from build123d import *

# Parameters (mm, degrees)
SKETCH1_W           = 13
SKETCH1_H           = 23
BOSS_EXTRUDE1_DEPTH = 23
CUT_EXTRUDE1_REACH  = 25
SKETCH1_3_W         = 12
SKETCH1_3_H         = 22
SKETCH2_W           = 13
SKETCH2_H           = 5.5
SKETCH2_R           = 1
BOSS_EXTRUDE2_DEPTH = 1
SKETCH4_W           = 8
SKETCH4_H           = 16
BOSS_EXTRUDE3_DEPTH = 10
CUT_EXTRUDE2_REACH  = 12.5
SKETCH5_W           = 14
SKETCH5_H           = 8
CUT_EXTRUDE3_REACH  = 22
SKETCH6_W           = 7
SKETCH6_H           = 9


with BuildPart() as part:
    # Sketch1 → Boss-Extrude1 (new body)
    with BuildSketch(Plane.XY):
        Rectangle(SKETCH1_W, SKETCH1_H)
    extrude(amount=BOSS_EXTRUDE1_DEPTH)

    # Sketch1_3 → Cut-Extrude1 (cut, up to next)
    with BuildSketch(Plane.XY, mode=Mode.PRIVATE) as cut_extrude1_sk1:
        Rectangle(SKETCH1_3_W, SKETCH1_3_H)
    cut_extrude1_tool1 = extrude(cut_extrude1_sk1.sketch, amount=CUT_EXTRUDE1_REACH, mode=Mode.PRIVATE) & part.part
    add(cut_extrude1_tool1.solids().sort_by_distance((0, 0, 0))[0], mode=Mode.SUBTRACT)

    # Sketch2 → Boss-Extrude2 (add)
    with BuildSketch(Plane.XY.offset(23)):
        with Locations((0, 14.25)):
            Rectangle(SKETCH2_W, SKETCH2_H)
        with Locations((0, 14.5)):
            Circle(SKETCH2_R, mode=Mode.SUBTRACT)
        with Locations((0, -14.25)):
            Rectangle(SKETCH2_W, SKETCH2_H)
        with Locations((0, -14.5)):
            Circle(SKETCH2_R, mode=Mode.SUBTRACT)
    extrude(amount=-BOSS_EXTRUDE2_DEPTH)

    # Sketch4 → Boss-Extrude3 (add)
    with BuildSketch(Plane(origin=(0, -11.5, 0), x_dir=(-1, 0, 0), z_dir=(0, -1, 0))):
        with Locations((0, -11)):
            Rectangle(SKETCH4_W, SKETCH4_H)
    extrude(amount=BOSS_EXTRUDE3_DEPTH)

    # Sketch5 → Cut-Extrude2 (cut, up to next)
    with BuildSketch(Plane(origin=(4, 0, 0), x_dir=(0, 0, -1), z_dir=(1, 0, 0)), mode=Mode.PRIVATE) as cut_extrude2_sk1:
        with Locations((-11, -16.5)):
            Rectangle(SKETCH5_W, SKETCH5_H)
    cut_extrude2_tool1 = extrude(cut_extrude2_sk1.sketch, amount=-CUT_EXTRUDE2_REACH, mode=Mode.PRIVATE) & part.part
    add(cut_extrude2_tool1.solids().sort_by_distance((4, -16.5, 11))[0], mode=Mode.SUBTRACT)

    # Sketch6 → Cut-Extrude3 (cut, up to next)
    with BuildSketch(Plane(origin=(0, 0, 3), x_dir=(-1, 0, 0), z_dir=(0, 0, -1)), mode=Mode.PRIVATE) as cut_extrude3_sk1:
        with Locations((0, -16.5)):
            Rectangle(SKETCH6_W, SKETCH6_H)
    cut_extrude3_tool1 = extrude(cut_extrude3_sk1.sketch, amount=-CUT_EXTRUDE3_REACH, mode=Mode.PRIVATE) & part.part
    add(cut_extrude3_tool1.solids().sort_by_distance((0, -16.5, 3))[0], mode=Mode.SUBTRACT)


solid = part.part
CAD build for the part. Positions are in the model's coordinates, mm. A direction names the side the tool comes from. Coordinates: 2 decimals unless noted, no trailing zeros. Write each loop counter-clockwise with the first axis right and the second up, starting at its lowest first coordinate (ties: lowest second). Pieces come first, ordered by that corner, then holes. Notation, with made-up numbers: M 55.25,-23 L 73.25,-23 A18 cw 73.25,-12 Z; hole C 53.5,36 d2. An arc over 180 degrees is marked long. Answer as a JSON object with one key per item and string values. Group by question number.
1) Wall check: line 1 (Y direction, x = 0, z = 22.3); line 2 (Y direction, x = 0.75, z = 17); line 3 (X direction, y = -2.5, z = 6.5). Give the ranges that are in metal, low to high. Write a range as from..to.
2) Saw through at A-A (z = 10). Write the cut outline in (x, y), plus the area to 3 significant figures.
3) Saw through at B-B (y = -16). Write the cut outline in (x, z), plus the area to 3 significant figures.
4) Tool access for faces 1 (the face through (0, 11.5, 11)), 2 (the face through (4, -12, 11)), 3 (the face through (-6, 0, 11)): list every direction of +Z, -Z, +X, -X, +Y, -Y with a clear straight run to the whole face (end or side of a thin tool).
5) Saw through at D-D (y = -2.5). Write the cut outline in (x, z).
6) Pin check, flat tips, straight feed: pin 1 Ø1.1 at (x, z) = (1, 22.5) entering from -Y; pin 2 Ø2 at (x, z) = (5, 6.5) entering from +Y; pin 3 Ø11 at (y, z) = (-18, 11.5) entering from -X. Stop position of each tip, or through.
7) Saw through at C-C (x = 0). Write the cut outline in (y, z), plus the area to 3 significant figures.
Values follow:
{
 "1": {"line 1": "y = -17..-15.5, -13.5..-11, 11..13.5, 15.5..17", "line 2": "y = -21.5..-21, -12..-11, 11..11.5", "line 3": "x = -6.5..-6, 6..6.5"},
 "2": {"outline": "M -6.5,-11.5 L -4,-11.5 L -4,-12.5 L -3.5,-12.5 L -3.5,-12 L 3.5,-12 L 3.5,-12.5 L 4,-12.5 L 4,-11.5 L 6.5,-11.5 L 6.5,11.5 L -6.5,11.5 Z; M -4,-21.5 L 4,-21.5 L 4,-20.5 L 3.5,-20.5 L 3.5,-21 L -3.5,-21 L -3.5,-20.5 L -4,-20.5 Z; hole M -6,-11 L 6,-11 L 6,11 L -6,11 Z", "area": "44.0 mm2"},
 "3": {"outline": "M -6.5,22 L 6.5,22 L 6.5,23 L -6.5,23 Z; M -4,3 L -3.5,3 L -3.5,4 L -4,4 Z; M -4,18 L -3.5,18 L -3.5,19 L -4,19 Z; M 3.5,3 L 4,3 L 4,4 L 3.5,4 Z; M 3.5,18 L 4,18 L 4,19 L 3.5,19 Z", "area": "15.0 mm2"},
 "4": {"face 1": "-Z, +X, -X, +Y", "face 2": "-Z, +X, -Y", "face 3": "+Z, -Z"},
 "5": {"outline": "M -6.5,0 L -6,0 L -6,23 L -6.5,23 Z; M 6,0 L 6.5,0 L 6.5,23 L 6,23 Z"},
 "6": {"pin 1": "stops at y = -17", "pin 2": "stops at y = 11.5", "pin 3": "stops at x = -4"},
 "7": {"outline": "M -21.5,3 L -21,3 L -21,19 L -21.5,19 Z; M -17,22 L -15.5,22 L -15.5,23 L -17,23 Z; M -13.5,22 L -11.5,22 L -11.5,19 L -12,19 L -12,3 L -11.5,3 L -11.5,0 L -11,0 L -11,23 L -13.5,23 Z; M 11,0 L 11.5,0 L 11.5,22 L 13.5,22 L 13.5,23 L 11,23 Z; M 15.5,22 L 17,22 L 17,23 L 15.5,23 Z", "area": "46.0 mm2"}
}
